```python
from build123d import *

# Parameters (mm, degrees)
ESBO_O1_R                 = 18.4
RESSALTO_EXTRUS_O1_DEPTH  = 24
ESBO_O2_R                 = 17.5
RESSALTO_EXTRUS_O2_DEPTH  = 30
ESBO_O3_R                 = 6
RESSALTO_EXTRUS_O3_DEPTH  = 6.5
ESBO_O4_R                 = 2.5
RESSALTO_EXTRUS_O4_DEPTH  = 15.5
ESBO_O5_R                 = 1.5
CORTE_EXTRUS_O1_DEPTH     = 10
ESBO_O6_R                 = 1
RESSALTO_EXTRUS_O5_DEPTH  = 2.5
ESBO_O8_R                 = 13.3
RESSALTO_EXTRUS_O7_DEPTH  = 1
ESBO_O9_R                 = 1
RESSALTO_EXTRUS_O8_DEPTH  = 5.5
ESBO_O10_R                = 9
RESSALTO_EXTRUS_O9_DEPTH  = 4
ESBO_O11_W                = 5.6
ESBO_O11_H                = 2
RESSALTO_EXTRUS_O10_DEPTH = 9
ESBO_O12_OUTSIDE_W        = 59.42
ESBO_O12_OUTSIDE_H        = 59.42
CORTE_EXTRUS_O2_DEPTH     = 10


with BuildPart() as part:
    # Esboço1 → Ressalto-extrusão1 (new body)
    with BuildSketch(Plane.XY):
        Circle(ESBO_O1_R)
    extrude(amount=RESSALTO_EXTRUS_O1_DEPTH)

    # Esboço2 → Ressalto-extrusão2 (add)
    with BuildSketch(Plane.XY.offset(24)):
        Circle(ESBO_O2_R)
    extrude(amount=RESSALTO_EXTRUS_O2_DEPTH)

    # Esboço3 → Ressalto-extrusão3 (add)
    with BuildSketch(Plane(origin=(0, 0, 0), x_dir=(-1, 0, 0), z_dir=(0, 0, -1))):
        with Locations((0, 7)):
            Circle(ESBO_O3_R)
    extrude(amount=RESSALTO_EXTRUS_O3_DEPTH)

    # Esboço4 → Ressalto-extrusão4 (add)
    with BuildSketch(Plane(origin=(0, 0, -6.5), x_dir=(-1, 0, 0), z_dir=(0, 0, -1))):
        with Locations((0, 7)):
            Circle(ESBO_O4_R)
    extrude(amount=RESSALTO_EXTRUS_O4_DEPTH)

    # Esboço5 → Corte-extrusão1 (cut)
    with BuildSketch(Plane(origin=(0, 0, 0), x_dir=(-1, 0, 0), z_dir=(0, 0, -1))):
        with Locations((7.485925154, 12.966002708)):
            Circle(ESBO_O5_R)
        with Locations((14.971850307, 0)):
            Circle(ESBO_O5_R)
        with Locations((7.485925154, -12.966002708)):
            Circle(ESBO_O5_R)
        with Locations((-7.485925154, -12.966002708)):
            Circle(ESBO_O5_R)
        with Locations((-14.971850307, 0)):
            Circle(ESBO_O5_R)
        with Locations((-7.485925154, 12.966002708)):
            Circle(ESBO_O5_R)
    extrude(amount=-CORTE_EXTRUS_O1_DEPTH, mode=Mode.SUBTRACT)

    # Esboço6 → Ressalto-extrusão5 (add)
    with BuildSketch(Plane.XY.offset(54)):
        Circle(ESBO_O6_R)
    extrude(amount=RESSALTO_EXTRUS_O5_DEPTH)

    # Esboço8 → Ressalto-extrusão7 (add)
    with BuildSketch(Plane.XY.offset(56.5)):
        Circle(ESBO_O8_R)
    extrude(amount=RESSALTO_EXTRUS_O7_DEPTH)

    # Esboço9 → Ressalto-extrusão8 (add)
    with BuildSketch(Plane.XY.offset(57.5)):
        Circle(ESBO_O9_R)
    extrude(amount=RESSALTO_EXTRUS_O8_DEPTH)

    # Esboço10 → Ressalto-extrusão9 (add)
    with BuildSketch(Plane.XY.offset(63)):
        Circle(ESBO_O10_R)
    extrude(amount=RESSALTO_EXTRUS_O9_DEPTH)

    # Esboço11 → Ressalto-extrusão10 (add)
    with BuildSketch(Plane.XY.offset(57.5)):
        with Locations((0, 10.3)):
            Rectangle(ESBO_O11_W, ESBO_O11_H)
    extrude(amount=RESSALTO_EXTRUS_O10_DEPTH)

    # Esboço12 outside → Corte-extrusão2 (cut)
    with BuildSketch(Plane(origin=(0, 0, -22), x_dir=(-1, 0, 0), z_dir=(0, 0, -1))):
        Rectangle(ESBO_O12_OUTSIDE_W, ESBO_O12_OUTSIDE_H)
        with BuildLine():
            Line((2, 8.5), (-2, 8.5))
            ThreePointArc((-2, 8.5), (0, 4.5), (2, 8.5))
        make_face(mode=Mode.SUBTRACT)
    extrude(amount=-CORTE_EXTRUS_O2_DEPTH, mode=Mode.SUBTRACT)


solid = part.part
```
Read the model definition and answer for the solid it produces. Units are mm, in the model's axes. A direction names the side the tool comes from. Give positions to 0.01 mm unless a question says otherwise; leave off trailing zeros. Write each loop counter-clockwise with the first axis right and the second up, starting at its lowest first coordinate (ties: lowest second). Pieces come first, ordered by that corner, then holes. Notation, with made-up numbers: M 82,7.5 L 114,7.5 A15 ccw 114,11.5 Z; hole C 74.25,85.25 d11. An arc over 180 degrees is marked long. Put each result on its own line as item: value. Start each with the question number.
1. The part is cut by section A-A, the plane z = 58.5. Give the vertices of the cut face in (x, y).
2. Each of these flat-tipped pins is pushed along its axis until it touches: pin 1 Ø5 at (x, z) = (-5.5, 30.5) entering from -Y; pin 2 Ø2 at (y, z) = (10, 62.5) entering from -X; pin 3 Ø8 at (x, y) = (-5.5, 2.5) entering from -Z. Where does it stop, or does it pass through?
3. Consider line 1 along Z through (x, y) = (-8, -3.5); line 2 along Z through (x, y) = (-2, 1.5); line 3 along Z through (x, y) = (-11.5, 4). Determine where each line is inside the solid, lowest interval first.
4. The part is cut by section C-C, the plane x = 8. Give the vertices of the cut face in (y, z).
5. Which of the six approach directions +Z, -Z, +X, -X, +Y, -Y give full straight-line access (tool end or side, diameter ignored) to faces 4 (the cylindrical face through (-1.15, 4.78, -14.14)), 5 (the cylindrical face through (-1.172, 8.923, 64.972)), 6 (the flat face through (0, 8.5, -17))?
6. The part is cut by section B-B, the plane y = -5.5. Give the vertices of the cut face in (x, z), and give its area (3 significant figures).
7. For a pull along Z with two mould halves and no side action, classify faces 1 (the cylindrical face through (0, -1, 55)), 2 (the cylindrical face through (6.8, -14.3, 4.9)), 3 (the flat face through (0, 0, 0)) as released by +Z, released by -Z, zero draft, split by the parting line, or undercut.
8. The part is cut by section D-D, the plane x = 12. Give the vertices of the cut face in (y, z), and give its area (3 significant figures).
Final values:
1. outline: M -2.8,9.3 L 2.8,9.3 L 2.8,11.3 L -2.8,11.3 Z; C 0,0 d2
2. pin 1: stops at y = -17.24
2. pin 2: stops at x = -2.8
2. pin 3: stops at z = -6.5
3. line 1: z = 0 to 54, 56.5 to 57.5, 63 to 67
3. line 2: z = -6.5 to 54, 56.5 to 57.5, 63 to 67
3. line 3: z = 0 to 54, 56.5 to 57.5
4. outline: M -16.57,0 L -14.38,0 L -14.38,10 L -11.56,10 L -11.56,0 L 11.56,0 L 11.56,10 L 14.38,10 L 14.38,0 L 16.57,0 L 16.57,24 L 15.56,24 L 15.56,54 L -15.56,54 L -15.56,24 L -16.57,24 Z; M -10.62,56.5 L 10.62,56.5 L 10.62,57.5 L -10.62,57.5 Z; M -4.12,63 L 4.12,63 L 4.12,67 L -4.12,67 Z
5. face 4: -Z
5. face 5: +Z
5. face 6: -Z, +X, -X, +Y
6. outline: M -17.56,0 L 17.56,0 L 17.56,24 L 16.61,24 L 16.61,54 L -16.61,54 L -16.61,24 L -17.56,24 Z; M -12.11,56.5 L 12.11,56.5 L 12.11,57.5 L -12.11,57.5 Z; M -7.12,63 L 7.12,63 L 7.12,67 L -7.12,67 Z
6. area: 1,920 mm²
7. face 1: undercut
7. face 2: zero draft
7. face 3: released by -Z
8. outline: M -13.95,0 L 13.95,0 L 13.95,24 L 12.74,24 L 12.74,54 L -12.74,54 L -12.74,24 L -13.95,24 Z; M -5.73,56.5 L 5.73,56.5 L 5.73,57.5 L -5.73,57.5 Z
8. area: 1,450 mm²
